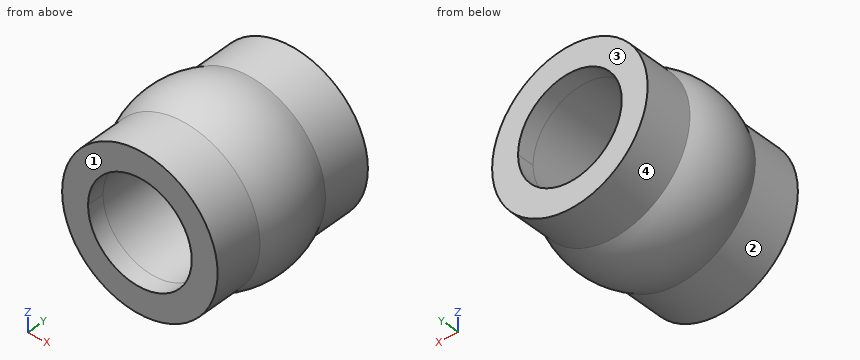
Autodesk Inventor part; units mm, degrees
ref_plane "YZ Plane" through (0, 0, 0) normal (1, 0, 0) x (0, 1, 0)
ref_plane "XZ Plane" through (0, 0, 0) normal (0, 1, 0) x (-1, 0, 0)
ref_plane "XY Plane" through (0, 0, 0) normal (0, 0, 1) x (1, 0, 0)
sketch "スケッチ1" plane through (0, 0, 0) normal (0, 0, 1) x (1, 0, 0)
  line L0 (0, 0) -> (0, 2.5)
  line L1 (0, 0) -> (0, -2.5)
  arc A0 (0, 2.5) -> (0, -2.5) centre (0, 0) ccw
  dimension "d0" = 2.5
  dimension "d1" = 2.5
  dimension "d2" = 2.5
revolve "回転1" add sketch "スケッチ1" angle 360 about axis through (0, 0, 0) along (0, 1, 0)
sketch "スケッチ2" plane through (0, 0, 0) normal (0, 1, 0) x (-1, 0, 0)
  circle A0 centre (0, 0) radius 1.5
  circle A1 centre (0, 0) radius 2.25
  dimension "d4" = 3
  dimension "d5" = 4.5
extrude "押し出し1" add sketch "スケッチ2" along normal mid plane 5
sketch "スケッチ3" plane through (0, 2.5, 0) normal (0, 1, 0) x (1, 0, 0)
  circle A0 centre (0, 0) radius 1.5
extrude "押し出し2" cut sketch "スケッチ3" against normal through all
properties part number "タミヤダンパー8" material "アセタール樹脂、黒"
For this review, take the finished solid that the model builds, in its own axes (mm). Face numbers are marked on the shaded views. A direction names the side the tool comes from. Round coordinates to 2 decimals unless told otherwise and drop trailing zeros. Write each loop counter-clockwise with the first axis right and the second up, starting at its lowest first coordinate (ties: lowest second). Pieces come first, ordered by that corner, then holes. Notation, with made-up numbers: (80.5, -21) - (127.5, -21) arc R13 cw to (127.5, 3) - close; hole circle Ø4 at (33.5, 54). An arc over 180 degrees is marked (long way). Use a Markdown table: item, result.
Q1. We need section A-A (x = 0). Give the boundary of the cut face in (y, z).
Derived:
| item | result |
|---|---|
| outline | (-2.5, -2.25) - (-1.09, -2.25) arc R2.5 ccw to (1.09, -2.25) - (2.5, -2.25) - (2.5, -1.5) - (-2.5, -1.5) - close; (-2.5, 1.5) - (2.5, 1.5) - (2.5, 2.25) - (1.09, 2.25) arc R2.5 ccw to (-1.09, 2.25) - (-2.5, 2.25) - close |
Q2. Machinability: for the marked faces 3 and 4, which of the approach directions +Z, -Z, +X, -X, +Y, -Y give a long, thin tool a straight path to every point of the face, cutting with its end or side? Answer none if there is none.
Derived:
| item | result |
|---|---|
| face 3 | +Z, -Z, +X, -X, +Y |
| face 4 | +Y |
Q3. We need section B-B (y = 1.35). Give the boundary of the cut face in (x, z), plus the area to 3 significant figures.
Derived:
| item | result |
|---|---|
| outline | circle Ø4.5 at (0, 0); hole circle Ø3 at (0, 0) |
| area | 8.84 mm2 |
Q4. Wall thickness on line 1 along Z through (x, y) = (0, 0.05); line 2 along Z through (x, y) = (0.1, 0.7): over which ranges is each line inside the solid? List them lowest first.
Derived:
| item | result |
|---|---|
| line 1 | z = -2.5 to -1.5, 1.5 to 2.5 |
| line 2 | z = -2.4 to -1.5, 1.5 to 2.4 |
Q5. The part is to be moulded in two halves that separate along Z. For the marked faces 1 and 2, say which applies: pulls with the +Z half, pulls with the -Z half, needs draft (parallel to the pull), parting line crosses it, or undercut.
Derived:
| item | result |
|---|---|
| face 1 | needs draft |
| face 2 | parting line crosses it |
Q6. We need section D-D (x = 0.95). Give the boundary of the cut face in (y, z).
Derived:
| item | result |
|---|---|
| outline | (-2.5, -2.04) - (-1.09, -2.04) arc R2.31 ccw to (1.09, -2.04) - (2.5, -2.04) - (2.5, -1.16) - (-2.5, -1.16) - close; (-2.5, 1.16) - (2.5, 1.16) - (2.5, 2.04) - (1.09, 2.04) arc R2.31 ccw to (-1.09, 2.04) - (-2.5, 2.04) - close |
Q7. We need section C-C (z = -2). Give the boundary of the cut face in (x, y), plus the area to 3 significant figures.
Derived:
| item | result |
|---|---|
| outline | (-1.03, -2.5) - (1.03, -2.5) - (1.03, -1.09) arc R1.5 ccw to (1.03, 1.09) - (1.03, 2.5) - (-1.03, 2.5) - (-1.03, 1.09) arc R1.5 ccw to (-1.03, -1.09) - close |
| area | 11.7 mm2 |
Q8. Clearance check with a flat-ended pin moving along its axis: pin 1 (1.5 mm diameter, centred on x = -1, y = -1, fed in from -Z). State where the tip first meets the part, or that it passes through.
Derived:
| item | result |
|---|---|
| pin 1 | stops at z = -2.41 |
